from build123d import *

# Parameters (mm, degrees)
SKETCH1_W           = 35.61
SKETCH1_H           = 20
BOSS_EXTRUDE1_DEPTH = 3
SKETCH3_R           = 1.5
CUT_EXTRUDE1_DEPTH  = 5
SKETCH7_W           = 15.61
SKETCH7_H           = 10
BOSS_EXTRUDE4_DEPTH = 30
BOSS_EXTRUDE5_DEPTH = 15.61
SKETCH9_R           = 1.5
CUT_EXTRUDE2_DEPTH  = 5


with BuildPart() as part:
    # Sketch1 → Boss-Extrude1 (new body)
    with BuildSketch(Plane(origin=(0, 0, 0), x_dir=(1, 0, 0), z_dir=(0, 1, 0))):
        with Locations((-8.436781609, 10.25)):
            Rectangle(SKETCH1_W, SKETCH1_H)
    extrude(amount=BOSS_EXTRUDE1_DEPTH)

    # Sketch3 → Cut-Extrude1 (cut)
    with BuildSketch(Plane.XZ):
        with Locations(Location((-20.484687418, -8.75, 0), (0, 0, 270))):
            Circle(SKETCH3_R)
        with Locations(Location((-8.434877213, -16.25, 0), (0, 0, 270))):
            Circle(SKETCH3_R)
        with Locations(Location((3.614932992, -8.75, 0), (0, 0, 270))):
            Circle(SKETCH3_R)
    extrude(amount=-CUT_EXTRUDE1_DEPTH, mode=Mode.SUBTRACT)

    # Sketch7 → Boss-Extrude4 (add)
    with BuildSketch(Plane(origin=(0, 3, 0), x_dir=(1, 0, 0), z_dir=(0, 1, 0))):
        with Locations((-8.436781609, 5.25)):
            Rectangle(SKETCH7_W, SKETCH7_H)
    extrude(amount=BOSS_EXTRUDE4_DEPTH)

    # Sketch8 → Boss-Extrude5 (add)
    with BuildSketch(Plane.ZY.offset(16.241781609)):
        Polygon((-10.25, 33), (-0.25, 50.320508076), (-0.25, 33), align=None)
    extrude(amount=-BOSS_EXTRUDE5_DEPTH)

    # Sketch9 → Cut-Extrude2 (cut)
    with BuildSketch(Plane(origin=(0, 12.688380194, -21.976919162), x_dir=(1, 0, 0), z_dir=(0, 0.4999999999999978, -0.8660254037844399))):
        with Locations(Location((-11.436781609, -33.453838325, 0), (0, 0, 270))):
            Circle(SKETCH9_R)
        with Locations(Location((-5.436781609, -33.453838325, 0), (0, 0, 270))):
            Circle(SKETCH9_R)
    extrude(amount=-CUT_EXTRUDE2_DEPTH, mode=Mode.SUBTRACT)


solid = part.part
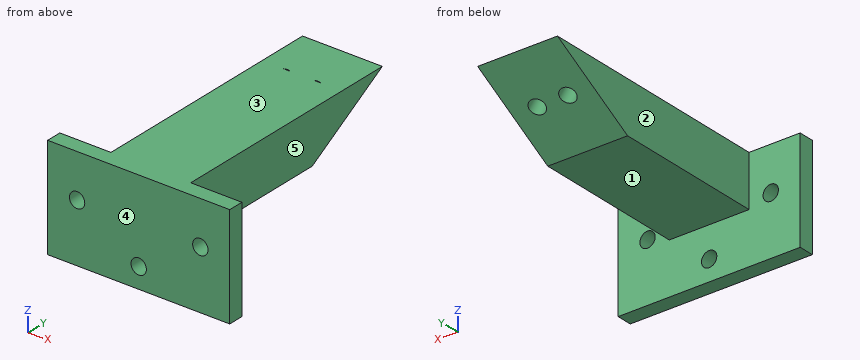
CAD build for the part. Positions are in the model's coordinates, mm. Face numbers are marked on the shaded views. A direction names the side the tool comes from. Give positions to 0.01 mm unless a question says otherwise; leave off trailing zeros. Order: outer loops, then holes, each group sorted by start corner. A loop starts at its lowest first (then second) coordinate and runs counter-clockwise, first axis right, second up. Notation, with made-up numbers: (-31.5, 11) - (21.5, 11) arc R7 cw to (21.5, 15) - close; hole circle Ø6 at (-31.75, -1). An arc over 180 degrees is marked (long way). Answer in a Markdown table with one row per item.
1. Tool access for the marked faces 1, 2, 3, 4 and 5: list every direction of +Z, -Z, +X, -X, +Y, -Y with a clear straight run to the whole face (end or side of a thin tool).
Data:
| item | result |
|---|---|
| face 1 | -Z, +X, -X, +Y |
| face 2 | +Z, -Z, -X, +Y |
| face 3 | +Z, +X, -X, +Y, -Y |
| face 4 | +Z, -Z, +X, -X, -Y |
| face 5 | +Z, -Z, +X, +Y |
2. Saw through at B-B, the plane z = -8.75. Give the cut face in (x, y).
Data:
| item | result |
|---|---|
| outline | (-26.24, 0) - (-21.98, 0) - (-21.98, 3) - (-26.24, 3) - close; (-18.98, 0) - (2.11, 0) - (2.11, 3) - (-0.63, 3) - (-0.63, 35.6) - (-16.24, 35.6) - (-16.24, 3) - (-18.98, 3) - close; (5.11, 0) - (9.37, 0) - (9.37, 3) - (5.11, 3) - close |
3. Saw through at A-A, the plane z = -16.25. Give the cut face in (x, y), plus the area to 3 significant figures.
Data:
| item | result |
|---|---|
| outline | (-26.24, 0) - (-9.93, 0) - (-9.93, 3) - (-26.24, 3) - close; (-6.93, 0) - (9.37, 0) - (9.37, 3) - (-6.93, 3) - close |
| area | 97.8 mm² |
4. Saw through at C-C, the plane x = 3. Give the cut face in (y, z).
Data:
| item | result |
|---|---|
| outline | (0, -20.25) - (3, -20.25) - (3, -10.12) - (0, -10.12) - close; (0, -7.38) - (3, -7.38) - (3, -0.25) - (0, -0.25) - close |
5. Saw through at D-D, the plane y = 25. Give the cut face in (x, z).
Data:
| item | result |
|---|---|
| outline | (-16.24, -10.25) - (-0.63, -10.25) - (-0.63, -0.25) - (-16.24, -0.25) - close |
6. Flat gauge pins, fed straight in: pin 1 (12.5 mm diameter, centred on x = -9.5, y = 21.5, fed in from -Z); pin 2 (1 mm diameter, centred on y = 25.5, z = -12, fed in from -X) (1 decimal); pin 3 (4 mm diameter, centred on x = 3.61, z = -8.75, fed in from +Y); pin 4 (5 mm diameter, centred on y = 29.5, z = -5.5, fed in from -X). Where does each tip first touch, or does it go through?
Data:
| item | result |
|---|---|
| pin 1 | stops at z = -10.25 |
| pin 2 | passes through |
| pin 3 | stops at y = 3 |
| pin 4 | stops at x = -16.24 |
7. Probe probe 1 along X at (y, z) = (2.45, -8.75); probe 2 along X at (y, z) = (41, -4); probe 3 along Z at (x, y) = (-6.5, 3.5). List the from-to ranges inside material, lowest first. Write a range as [from, to].
Data:
| item | result |
|---|---|
| probe 1 | x = [-26.24, -21.98], [-18.98, 2.11], [5.11, 9.37] |
| probe 2 | x = [-16.24, -12.94], [-9.94, -6.94], [-3.94, -0.63] |
| probe 3 | z = [-10.25, -0.25] |
